Here's how the part is built. I have some questions about the finished solid (model axes, mm). Round coordinates to 2 decimals unless told otherwise and drop trailing zeros. Loops run counter-clockwise (first coordinate to the right, second up) from the corner with the lowest first, then second, coordinate; pieces in that order, holes last. Notation, with made-up numbers: (87.25, -38) - (98.25, -38) arc R19 cw to (98.25, -9) - close; hole circle Ø5 at (37, -24). An arc over 180 degrees is marked (long way). Return JSON: item names as keys, results as strings. Group by question number.
```python
from build123d import *

# Parameters (mm, degrees)
BOSS_EXTRUDE1_DEPTH    = 3.175
F_10_CLEARANCE_HOLE1_D = 4.9784
BOSS_EXTRUDE2_DEPTH    = 4.7625
F_8_CLEARANCE_HOLE1_D  = 4.3053


with BuildPart() as part:
    # Sketch1 → Boss-Extrude1 (new body)
    with BuildSketch(Plane.XY):
        Polygon((-254.000000508, -12.7), (-266.700000508, -12.7), (-266.700000508, 57.15), (-254.000000508, 57.15), (-222.250000508, 57.15), (-203.200000508, 38.1), (-203.200000508, 12.7), (-203.200000508, -12.7), align=None)
    extrude(amount=BOSS_EXTRUDE1_DEPTH)

    # #10 Clearance Hole1 (through all)
    with Locations(Plane.XY.offset(3.175)):
        with Locations((-260.311771093, 50.798866939), (-260.350000508, 25.4), (-260.350000508, 0), (-241.300000508, 0), (-215.900000508, 0)):
            Hole(F_10_CLEARANCE_HOLE1_D / 2)

    # Sketch5 → Boss-Extrude2 (add)
    with BuildSketch(Plane.XY.offset(3.175)):
        Polygon((-222.250000508, 57.15), (-234.950000508, 57.15), (-234.950000508, 12.7), (-222.250000508, 12.7), (-222.250000508, 50.8), align=None)
    extrude(amount=BOSS_EXTRUDE2_DEPTH)

    # #8 Clearance Hole1 (through all)
    with Locations(Plane.XY.offset(7.9375)):
        with Locations((-228.600000508, 42.8625), (-228.600000508, 52.3875), (-228.600000508, 33.3375), (-228.600000508, 23.8125)):
            Hole(F_8_CLEARANCE_HOLE1_D / 2)


solid = part.part
```
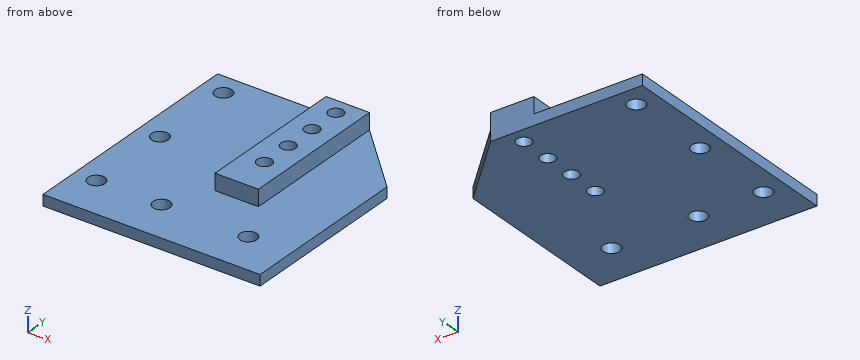
Q1. Please list where these lines run through material, in increasing order: line 1 (Y direction, x = -228.6, z = 4.75); line 2 (Y direction, x = -241.3, z = 1.1); line 3 (Z direction, x = -254, y = 6) (3 decimals).
Q2. Imagine slicing it at D-D, the plane x = -260.35. List the corners of the cut face in (y, z) for me (3 decimals).
Q3. Imagine slicing it at C-C, the plane z = 5. List the corners of the cut face in (x, y) for me.
Q4. Will these pins go through, and if not, where does the flat tip stop? pin 1 Ø1.5 at (x, y) = (-247.5, -4) entering from +Z (3 decimals); pin 2 Ø4 at (y, z) = (43.5, 6.5) entering from -X; pin 3 Ø1.4 at (x, z) = (-228.5, 5.5) entering from -Y.
Q5. Imagine slicing it at A-A, the plane x = -215.9. List the corners of the cut face in (y, z) for me (3 decimals).
Output values:
{
 "1": {"line 1": "y = 12.7 to 21.66, 25.97 to 31.18, 35.49 to 40.71, 45.02 to 50.23, 54.54 to 57.15", "line 2": "y = -12.7 to -2.49, 2.49 to 57.15", "line 3": "z = 0 to 3.175"},
 "2": {"outline": "(-12.7, 0) - (-2.489, 0) - (-2.489, 3.175) - (-12.7, 3.175) - close; (2.489, 0) - (22.911, 0) - (22.911, 3.175) - (2.489, 3.175) - close; (27.889, 0) - (48.31, 0) - (48.31, 3.175) - (27.889, 3.175) - close; (53.288, 0) - (57.15, 0) - (57.15, 3.175) - (53.288, 3.175) - close"},
 "3": {"outline": "(-234.95, 12.7) - (-222.25, 12.7) - (-222.25, 57.15) - (-234.95, 57.15) - close; hole circle Ø4.31 at (-228.6, 23.81); hole circle Ø4.31 at (-228.6, 33.34); hole circle Ø4.31 at (-228.6, 42.86); hole circle Ø4.31 at (-228.6, 52.39)"},
 "4": {"pin 1": "stops at z = 3.175", "pin 2": "stops at x = -234.95", "pin 3": "stops at y = 12.7"},
 "5": {"outline": "(-12.7, 0) - (-2.489, 0) - (-2.489, 3.175) - (-12.7, 3.175) - close; (2.489, 0) - (50.8, 0) - (50.8, 3.175) - (2.489, 3.175) - close"}
}
